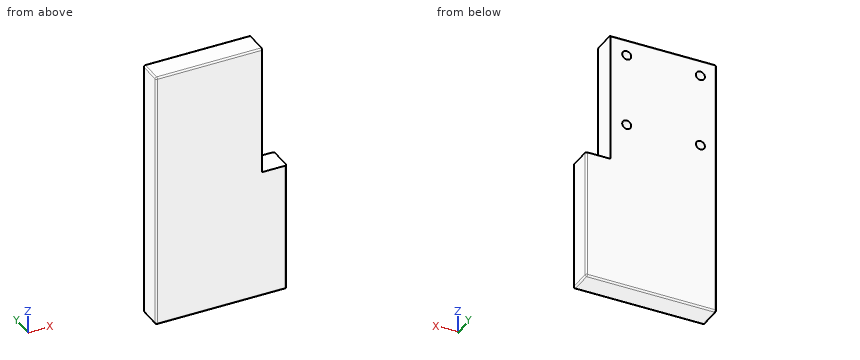
from build123d import *

# Parameters (mm, degrees)
F0_W     = 160
F0_H     = 30
F1_DEPTH = 160
F2_R     = 2
F3_W     = 28
F3_H     = 158
F4_DEPTH = 30.001
F3_R     = 5.5
F5_DEPTH = 15


with BuildPart() as f1:
    # F0 (on Top) → F1 (new body, symmetric)
    with BuildSketch(Plane.XY):
        Rectangle(F0_W, F0_H)
    extrude(amount=F1_DEPTH, both=True)

    # F2
    f2_edges = [f1.edges().sort_by_distance(p)[0] for p in [
        (0, -15, -160),
        (80, -15, 0),
        (0, -15, 160),
        (-80, -15, 0),
        (80, 15, 0),
        (0, 15, -160),
        (-80, 15, 0),
        (0, 15, 160),
        (80, 0, 160),
        (-80, 0, 160),
        (80, 0, -160),
        (-80, 0, -160),
    ]]
    fillet(f2_edges, radius=F2_R)

    # F3 (on face) → F4 (cut, through all)
    with BuildSketch(Plane(origin=(0, 15, 0), x_dir=(-1, 0, 0), z_dir=(0, 1, 0))):
        with Locations((-64, 79)):
            Rectangle(F3_W, F3_H)
        Polygon((-80, 0), (-78, 0), (-78, 158), (-50, 158), (-50, 160), (-80, 160), align=None)
    extrude(amount=-F4_DEPTH, mode=Mode.SUBTRACT)

    # F3 (on face) → F5 (cut)
    with BuildSketch(Plane(origin=(0, 15, 0), x_dir=(-1, 0, 0), z_dir=(0, 1, 0))):
        with Locations((60, 140)):
            Circle(F3_R)
        with Locations((-30, 140)):
            Circle(F3_R)
        with Locations((-30, 50)):
            Circle(F3_R)
        with Locations((60, 50)):
            Circle(F3_R)
    extrude(amount=-F5_DEPTH, mode=Mode.SUBTRACT)


solid = f1.part
Can you work these out from the model? Positions are in its coordinate system, mm. Coordinates: 2 decimals unless noted, no trailing zeros. Loops run counter-clockwise (first coordinate to the right, second up) from the corner with the lowest first, then second, coordinate; pieces in that order, holes last. Notation, with made-up numbers: (-30.5, 67) - (-18.5, 67) arc R18 cw to (-18.5, 100) - close; hole circle Ø6 at (8.5, 22). An arc over 180 degrees is marked (long way). Put each result on its own line as item: value. Start each with the question number.
Item 1: If I drill on line 1 along Z through (x, y) = (30, 4); line 2 along Z through (x, y) = (25, 3); line 3 along X through (y, z) = (-2.5, 47), over which ranges is the centre line in solid material (lowest first)?
Item 2: For pin 1 (3.5 mm diameter, centred on x = 30.5, z = 51.5, fed in from +Y); pin 2 (15 mm diameter, centred on y = -4, z = 103.5, fed in from +X), each with a flat end and sliding along its axis, tell me the tip position at first contact or that it passes through.
Item 3: Suppose I cut it at B-B (z = 50). Please give me the cut outline in (x, y), and give its area (3 significant figures).
Item 4: Suppose I cut it at A-A (x = -60). Please give me the cut outline in (y, z), and give its area (3 significant figures).
Item 5: Suppose I cut it at D-D (z = 123.5). Please give me the cut outline in (x, y).
Item 6: Suppose I cut it at C-C (y = -5.75). Please give me the cut outline in (x, z).
Here are the results:
1. line 1: -160 to 44.5, 55.5 to 134.5, 145.5 to 160
1. line 2: -160 to 47.71, 52.29 to 137.71, 142.29 to 160
1. line 3: -80 to 50
2. pin 1: y = 0
2. pin 2: x = 50
3. outline: (-80, -13) arc R2 ccw to (-78, -15) - (50, -15) - (50, 15) - (35.5, 15) - (35.5, 0) - (24.5, 0) - (24.5, 15) - (-54.5, 15) - (-54.5, 0) - (-65.5, 0) - (-65.5, 15) - (-78, 15) arc R2 ccw to (-80, 13) - close
3. area: 3,570 mm²
4. outline: (-15, -158) arc R2 ccw to (-13, -160) - (13, -160) arc R2 ccw to (15, -158) - (15, 44.5) - (0, 44.5) - (0, 55.5) - (15, 55.5) - (15, 134.5) - (0, 134.5) - (0, 145.5) - (15, 145.5) - (15, 158) arc R2 ccw to (13, 160) - (-13, 160) arc R2 ccw to (-15, 158) - close
4. area: 9,270 mm²
5. outline: (-80, -13) arc R2 ccw to (-78, -15) - (50, -15) - (50, 15) - (-78, 15) arc R2 ccw to (-80, 13) - close
6. outline: (-80, -158) arc R2 ccw to (-78, -160) - (78, -160) arc R2 ccw to (80, -158) - (80, 0) - (50, 0) - (50, 160) - (-78, 160) arc R2 ccw to (-80, 158) - close
